Model file for the job. Use its own axes, mm. A direction names the side the tool comes from. Coordinates: 2 decimals unless noted, no trailing zeros. Write each loop counter-clockwise with the first axis right and the second up, starting at its lowest first coordinate (ties: lowest second). Pieces come first, ordered by that corner, then holes. Notation, with made-up numbers: M -19.5,-0.75 L 32.5,-0.75 A21 ccw 32.5,23.25 Z; hole C 0,54.25 d1. An arc over 180 degrees is marked long. One line per question, with ' | ' between items. Start each with the question number.
(1) Cut at A-A (x = 7). Write the cut outline in (y, z), plus the area to 3 significant figures.
(2) Tool access for faces 1 (the face through (0, 20, 192)), 2 (the face through (2, 22, 192)): list every direction of +Z, -Z, +X, -X, +Y, -Y with a clear straight run to the whole face (end or side of a thin tool).
(3) Cut at B-B (z = 381). Write the cut outline in (x, y), plus the area to 3 significant figures.
(4) Cut at C-C (y = 20). Write the cut outline in (x, z), plus the area to 3 significant figures.
(5) Wall check: probe 1 along Y at (x, z) = (0.85, 404); probe 2 along X at (y, z) = (23, 123); probe 3 along Y at (x, z) = (22.75, 101). Give the ranges that are in metal, low to high.
(6) Two-plate mould, pull along Y, no slides. Class faces 3 (the face through (16, 7.602, 192)), 4 (the face through (8, 7, -20)), 5 (the face through (15, 5.602, 192)): +Y half, -Y half, draft (parallel to the pull), parting line (faces both ways), or undercut.
(7) Flat gauge pins, fed straight in: pin 1 Ø12 at (y, z) = (16.5, 230) entering from +X; pin 2 Ø6 at (x, y) = (7, 8.5) entering from +Z. Where does each tip first touch, or does it go through?
from build123d import *

# Parameters (mm, degrees)
BOSS_EXTRUDE1_DEPTH      = 410
BOSS_EXTRUDE1_DEPTH_BACK = 20
F_3_0_3_DIAMETER_HOLE2_D = 3
F_3_0_3_DIAMETER_HOLE4_D = 3


with BuildPart() as part:
    # Sketch1 → Boss-Extrude1 (new, two sides: drawn at the far end of the back side and taken through both)
    with BuildSketch(Plane.XY.offset(-BOSS_EXTRUDE1_DEPTH_BACK)):
        Polygon((0, 5.602318429), (0, 35.602318429), (2, 35.602318429), (2, 7.602318429), (30, 7.602318429), (30, 5.602318429), align=None)
    extrude(amount=BOSS_EXTRUDE1_DEPTH + BOSS_EXTRUDE1_DEPTH_BACK)

    # Ø3.0 (3) Diameter Hole2 (through all)
    with Locations(Plane(origin=(0, 369.009951222, 221.32004832), x_dir=(0, 0, -1), z_dir=(-1, 0, 0))):
        with Locations((235.32004832, 341.407632793), (235.32004832, 355.407632793)):
            Hole(F_3_0_3_DIAMETER_HOLE2_D / 2)

    # Ø3.0 (3) Diameter Hole4 (through all)
    with Locations(Plane(origin=(2, 369.009951222, 221.32004832), x_dir=(0, 0, 1), z_dir=(1, 0, 0))):
        with Locations((182.67995168, 355.407632793), (182.67995168, 341.407632793)):
            Hole(F_3_0_3_DIAMETER_HOLE4_D / 2)


solid = part.part
Filled in:
1) outline: M 5.6,-20 L 7.6,-20 L 7.6,410 L 5.6,410 Z | area: 860 mm²
2) face 1: +Z, -Z, -X, +Y, -Y | face 2: +Z, -Z, +X, +Y
3) outline: M 0,5.6 L 30,5.6 L 30,7.6 L 2,7.6 L 2,35.6 L 0,35.6 Z | area: 116 mm²
4) outline: M 0,-20 L 2,-20 L 2,410 L 0,410 Z | area: 860 mm²
5) probe 1: 5.6 to 12.1, 15.1 to 26.1, 29.1 to 35.6 | probe 2: 0 to 2 | probe 3: 5.6 to 7.6
6) face 3: +Y half | face 4: draft | face 5: -Y half
7) pin 1: x = 2 | pin 2: z = 410
